Part model, mm, in its own coordinate system. A direction names the side the tool comes from. Give positions to 0.01 mm unless a question says otherwise; leave off trailing zeros. Write each loop counter-clockwise with the first axis right and the second up, starting at its lowest first coordinate (ties: lowest second). Pieces come first, ordered by that corner, then holes. Notation, with made-up numbers: (47.25, -20) - (105.25, -20) arc R19 ccw to (105.25, 17) - close; hole circle Ø8 at (43, -36.5). An arc over 180 degrees is marked (long way). Answer in a Markdown table with one row per item. Add a question column.
1. Band-saw the part on B-B on x = 70.5. Write the cut outline in (y, z).
2. Band-saw the part on C-C on y = 16. Write the cut outline in (x, z), plus the area to 3 significant figures.
3. Drop flat-ended pins along their axis: pin 1 Ø2 at (y, z) = (-4, -8) entering from -X; pin 2 Ø8 at (y, z) = (-18.5, 0) entering from +X; pin 3 Ø8 at (x, z) = (90.5, 3.5) entering from +Y. Give the stop position or say it passes through.
4. Which spindle directions (+Z, -Z, +X, -X, +Y, -Y) get a long thin tool onto all of the face, cutting with end or side? Do faces 1 (the cylindrical face through (86.21, 42.84, -0.14)), 2 (the flat face through (59.735, 35.027, -0.14)). Say none if no direction does.
5. Probe line 1 along Y through (x, z) = (96, 2.75); line 2 along X through (y, z) = (43.5, 4.5); line 3 along Y through (x, z) = (95, -5.5). List the from-to ranges inside material, lowest first.
6. Band-saw the part on A-A on z = 5. Write the cut outline in (x, y), plus the area to 3 significant figures.
7. Pull direction X, two halves, no side cores. Call faces 3 (the cylindrical face through (39.436, -3.715, 0.14)), 4 (the flat face through (50, 18, 10)), 5 (the flat face through (0, -31, 0)), 6 (the cylindrical face through (93.678, 22.604, 0.14)): released by +X, released by -X, zero draft, split by the parting line, or undercut.
```python
from build123d import *

# Parameters (mm, degrees)
F0_R          = 10
F1_DEPTH      = 10
F1_DEPTH_BACK = 10
F2_R          = 20
F3_R          = 10


with BuildPart() as f1:
    # F0 (on Top) → F1 (new body, two sides)
    with BuildSketch(Plane.XY) as f1_sk:
        with BuildLine():
            ThreePointArc((0, 25), (25, 0), (0, -25))
            Line((0, -25), (0, -37))
            ThreePointArc((0, -37), (25.050639293, -27.2298635878), (36.8716481479, -3.0792146493))
            Line((36.8716481479, -3.0792146493), (94.1099400271, 23.6114391937))
            ThreePointArc((94.1099400271, 23.6114391937), (117.4615775982, 42.7525179157), (87.2695371606, 42.4052916094))
            Line((87.2695371606, 42.4052916094), (26.2660401482, 26.0594538495))
            ThreePointArc((26.2660401482, 26.0594538495), (14.2267390426, 34.1555251199), (0, 37))
            Line((0, 37), (0, 25))
        make_face()
        with Locations((102.4264956657, 37.2801956225)):
            Circle(F0_R, mode=Mode.SUBTRACT)
    extrude(amount=-F1_DEPTH)
    extrude(f1_sk.sketch, amount=F1_DEPTH_BACK)

    # F2
    f2_edges = [f1.edges().sort_by_distance(p)[0] for p in [
        (26.26604, 26.059454, 0),
        (36.871648, -3.079215, 0),
    ]]
    fillet(f2_edges, radius=F2_R)

    # F3
    f3_edges = [f1.edges().sort_by_distance(p)[0] for p in [
        (87.269537, 42.405292, 0),
        (94.10994, 23.611439, 0),
    ]]
    fillet(f3_edges, radius=F3_R)


solid = f1.part
```
Values:
| question | item | result |
|---|---|---|
| 1 | outline | (12.6, -10) - (37.91, -10) - (37.91, 10) - (12.6, 10) - close |
| 2 | outline | (19.21, -10) - (77.79, -10) - (77.79, 10) - (19.21, 10) - close |
| 2 | area | 1,170 mm² |
| 3 | pin 1 | stops at x = 24.49 |
| 3 | pin 2 | stops at x = 34.04 |
| 3 | pin 3 | stops at y = 51.18 |
| 4 | face 1 | +Z, -Z, -X, +Y |
| 4 | face 2 | +Z, -Z, +Y |
| 5 | line 1 | y = 22.45 to 29.62, 44.94 to 51.93 |
| 5 | line 2 | x = 87.01 to 94.6, 110.26 to 117.17 |
| 5 | line 3 | y = 22.59 to 30.58, 43.98 to 51.45 |
| 6 | outline | (0, -37) arc R37 ccw to (35.32, -11.01) arc R20 cw to (45.96, 1.16) - (89.97, 21.68) arc R10 cw to (97.36, 22.1) arc R16 ccw (long way) to (88.79, 45.65) arc R10 cw to (82.86, 41.22) - (35.96, 28.66) arc R20 cw to (19.98, 31.14) arc R37 ccw to (0, 37) - (0, 25) arc R25 cw to (0, -25) - close; hole circle Ø20 at (102.43, 37.28) |
| 6 | area | 3,180 mm² |
| 7 | face 3 | released by +X |
| 7 | face 4 | zero draft |
| 7 | face 5 | released by -X |
| 7 | face 6 | undercut |
